Autodesk Inventor part; units mm, degrees
ref_plane "YZ Plane" through (0, 0, 0) normal (1, 0, 0) x (0, 1, 0)
ref_plane "XZ Plane" through (0, 0, 0) normal (0, 1, 0) x (-1, 0, 0)
ref_plane "XY Plane" through (0, 0, 0) normal (0, 0, 1) x (1, 0, 0)
sketch "Sketch1" plane through (0, 0, 0) normal (0, 0, 1) x (1, 0, 0)
  line L0 (-13.4502, 9.4461) -> (-471.2502, 9.4461)
  line L1 (-471.2502, 9.4461) -> (-471.2502, -295.3539)
  line L2 (-471.2502, -295.3539) -> (-13.4502, -295.3539)
  line L3 (-13.4502, -295.3539) -> (-13.4502, 9.4461)
  point P0 (0, 0)
  dimension "d0" = 457.8
  dimension "d1" = 304.8
extrude "Extrusion1" add sketch "Sketch1" along normal blind 457
sketch "Sketch2" plane through (-471.2502, 9.4461, 0) normal (0, 1, 0) x (1, 0, 0)
  line L0 (12.104, -443.504) -> (442.7261, -443.504)
  line L1 (442.7261, -443.504) -> (442.7261, -12.8819)
  line L2 (442.7261, -12.8819) -> (12.104, -12.8819)
  line L3 (12.104, -12.8819) -> (12.104, -443.504)
  point P0 (471.2502, 0)
extrude "Extrusion2" cut sketch "Sketch2" against normal blind 300
sketch "Sketch3" plane through (-13.4502, -295.3539, 0) normal (1, 0, 0) x (0, 0, -1)
  circle A0 centre (-248.4802, 267.8138) radius 4
  point P0 (0, 295.3539)
  dimension "d6" = 8
extrude "Extrusion3" add sketch "Sketch3" along normal blind 15
properties part number "outerbox"
Could you check a few things on this model? Use its own coordinates, in mm. A direction names the side the tool comes from. Coordinates: 2 decimals unless noted, no trailing zeros. Order: outer loops, then holes, each group sorted by start corner. A loop starts at its lowest first (then second) coordinate and runs counter-clockwise, first axis right, second up. Notation, with made-up numbers: (-28.5, -22) -> (8.5, -22) arc R34 cw to (8.5, 11) -> close; hole circle Ø1 at (78, -15.75). An arc over 180 degrees is marked (long way). One line per item, written item: value. Start each with the question number.
1) Imagine slicing it at B-B on x = -295. List the corners of the cut face in (y, z) for me.
2) We'd pull the mould along X, two halves only. Please class faces 1 (the flat face through (-471.25, -141, 225)), 2 (the flat face through (-246, -295.354, 225)), 3 (the flat face through (-28.524, -138, 231)): +X half, -X half, draft (parallel to the pull), parting line (faces both ways), or undercut.
3) If I drill on L1, parallel to X at y = -198, z = 243.5; L2, parallel to Z at x = -196.5, y = -40; L3, parallel to Y at x = -379, z = 141.5, over which ranges is the centre line in solid material (lowest first)? Write a range as [from, to].
4) I'm going to push flat-ended pins straight in: pin 1 (4 mm diameter, centred on x = -118.5, y = -194, fed in from -Z); pin 2 (4 mm diameter, centred on y = -21, z = 397.5, fed in from +X). Where does each tip first touch, or does it pass through?
5) Imagine slicing it at C-C on z = 412. List the corners of the cut face in (x, y) for me, plus the area to 3 significant figures.
6) Which directions (+Z, -Z, +X, -X, +Y, -Y) give clear straight access to the entire face, cutting with the end or side of a thin tool? Please do faces 4 (the flat face through (-246, -141, 457)), 5 (the flat face through (-247, -138, 443.504)).
7) Imagine slicing it at A-A on y = -180. List the corners of the cut face in (x, z) for me.
Answer list:
1. outline: (-295.35, 0) -> (9.45, 0) -> (9.45, 12.88) -> (-290.55, 12.88) -> (-290.55, 443.5) -> (9.45, 443.5) -> (9.45, 457) -> (-295.35, 457) -> close
2. face 1: -X half
2. face 2: draft
2. face 3: undercut
3. L1: x = [-471.25, -459.15], [-28.52, -13.45]
3. L2: z = [0, 12.88], [443.5, 457]
3. L3: y = [-295.35, -290.55]
4. pin 1: stops at z = 0
4. pin 2: stops at x = -13.45
5. outline: (-471.25, -295.35) -> (-13.45, -295.35) -> (-13.45, 9.45) -> (-28.52, 9.45) -> (-28.52, -290.55) -> (-459.15, -290.55) -> (-459.15, 9.45) -> (-471.25, 9.45) -> close
5. area: 10,400 mm2
6. face 4: +Z, +X, -X, +Y, -Y
6. face 5: +Y
7. outline: (-471.25, 0) -> (-13.45, 0) -> (-13.45, 457) -> (-471.25, 457) -> close; hole (-459.15, 12.88) -> (-28.52, 12.88) -> (-28.52, 443.5) -> (-459.15, 443.5) -> close
